Could you check a few things on this drawing? It's one solid part, dimensions in mm from its lowest x, y, z. Give positions to 0.01 mm unless a question says otherwise; leave off trailing zeros. Order: outer loops, then holes, each group sorted by start corner. A loop starts at its lowest first (then second) coordinate and runs counter-clockwise, first axis right, second up.
Item 1: If I drill on line 1 along X through (y, z) = (15, 5); line 2 along Y through (x, z) = (5, 1.65); line 3 along Y through (x, z) = (5, 0.9), over which ranges is the centre line in solid material (lowest first)?
Item 2: I want a section at D-D, the plane y = 45.5. Write out the boundary of the cut face in (x, z).
Item 3: I want a section at A-A, the plane y = 5. Write out the boundary of the cut face in (x, z).
Item 4: I'm going to push flat-ended pins straight in: pin 1 Ø1.5 at (x, z) = (2, 3.5) entering from +Y; pin 2 Ø1 at (y, z) = (34, 15.5) entering from +X; pin 3 Ø3 at (x, z) = (5, 11) entering from -Y. Where does each tip first touch, or does it pass through?
Item 5: I want a section at C-C, the plane z = 11.5. Write out the boundary of the cut face in (x, y).
Item 6: I want a section at B-B, the plane x = 4. Write out the boundary of the cut face in (y, z), then the cut area to 3 significant figures.
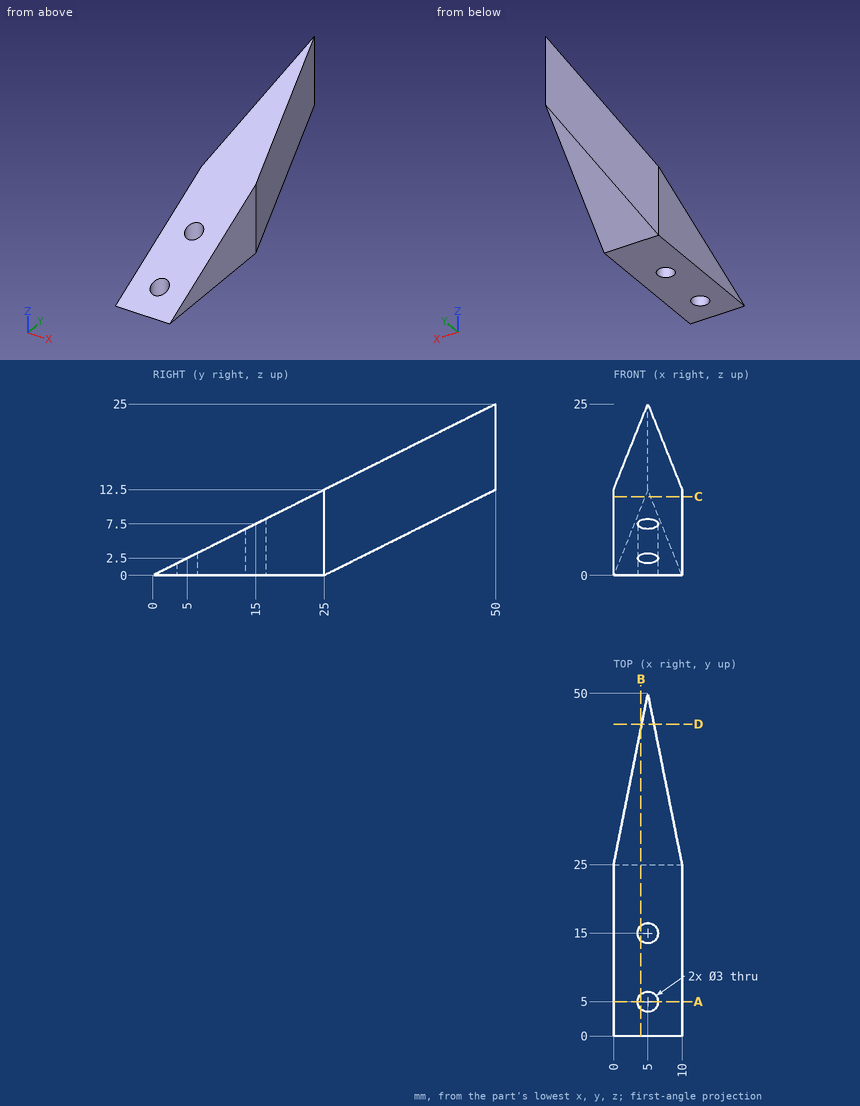
Results list:
1. line 1: x = 0 to 3.5, 6.5 to 10
1. line 2: y = 3.3 to 3.5, 6.5 to 13.5, 16.5 to 28.3
1. line 3: y = 1.8 to 3.5, 6.5 to 13.5, 16.5 to 26.8
2. outline: (4.1, 10.25) - (5.9, 10.25) - (5.9, 22.75) - (4.1, 22.75) - close
3. outline: (0, 0) - (3.5, 0) - (3.5, 2.5) - (0, 2.5) - close; (6.5, 0) - (10, 0) - (10, 2.5) - (6.5, 2.5) - close
4. pin 1: stops at y = 33.5
4. pin 2: stops at x = 8.3
4. pin 3: stops at y = 19
5. outline: (0, 23) - (10, 23) - (10, 25) - (5.4, 48) - (4.6, 48) - (0, 25) - close
6. outline: (0, 0) - (3.88, 0) - (3.88, 1.94) - close; (6.12, 0) - (13.88, 0) - (13.88, 6.94) - (6.12, 3.06) - close; (16.12, 0) - (25, 0) - (45, 10) - (45, 22.5) - (16.12, 8.06) - close
6. area: 384 mm2
